Part model, mm, in its own coordinate system. A direction names the side the tool comes from. Give positions to 0.01 mm unless a question says otherwise; leave off trailing zeros. Write each loop counter-clockwise with the first axis right and the second up, starting at its lowest first coordinate (ties: lowest second). Pieces come first, ordered by that corner, then holes.
from build123d import *

# Parameters (mm, degrees)
SKETCH_1_R          = 1.025
EXTRUDE_1_DEPTH     = 2.5
EXTRUDE_3_DEPTH     = 2.5
EXTRUDE_2_DEPTH     = 2.5
FILLET_1_R          = 4
CUT_EXTRUDE_1_DEPTH = 2.5
FILLET_3_R          = 1
FILLET_4_R          = 2


with BuildPart() as part:
    # 草图1 → 凸台-拉伸1 (new body)
    with BuildSketch(Plane(origin=(0, 0, 0), x_dir=(1, 0, 0), z_dir=(0, 1, 0))):
        with BuildLine():
            Line((0, 4), (30, 4))
            ThreePointArc((30, 4), (34, 0), (30, -4))
            Line((30, -4), (0, -4))
            ThreePointArc((0, -4), (-4, 0), (0, 4))
        make_face()
        with Locations(Location((30, 0, 0), (0, 0, 270))):
            Circle(SKETCH_1_R, mode=Mode.SUBTRACT)
        with BuildLine():
            Line((0, 1.6), (20, 1.6))
            ThreePointArc((20, 1.6), (21.6, 0), (20, -1.6))
            Line((20, -1.6), (0, -1.6))
            ThreePointArc((0, -1.6), (-1.6, 0), (0, 1.6))
        make_face(mode=Mode.SUBTRACT)
    extrude(amount=EXTRUDE_1_DEPTH)

    # 草图4 → 凸台-拉伸3 (add)
    with BuildSketch(Plane(origin=(0, 0, 0), x_dir=(1, 0, 0), z_dir=(0, 1, 0))):
        with BuildLine():
            Line((35, 4), (30, 4))
            ThreePointArc((30, 4), (34, 0), (30, -4))
            Line((30, -4), (35, -4))
            Line((35, -4), (35, 4))
        make_face()
    extrude(amount=EXTRUDE_3_DEPTH)

    # 草图2 → 凸台-拉伸2 (add)
    with BuildSketch(Plane.XZ):
        with BuildLine():
            Line((-4, 6.7), (-4, 0))
            ThreePointArc((-4, 0), (-2.828427125, 2.828427125), (0, 4))
            Line((0, 4), (33.541672043, 4))
            ThreePointArc((33.541672043, 4), (33.13675384, 5.32310053), (33, 6.7))
            ThreePointArc((33, 6.7), (14.5, 5.554795019), (-4, 6.7))
        make_face()
    extrude(amount=-EXTRUDE_2_DEPTH)

    # 圆角1
    fillet_1_edges = [part.edges().sort_by_distance(p)[0] for p in [
        (-4, 1.25, 6.7),
    ]]
    fillet(fillet_1_edges, radius=FILLET_1_R)

    # 草图5 → 切除-拉伸1 (cut)
    with BuildSketch(Plane(origin=(0, 2.5, 0), x_dir=(1, 0, 0), z_dir=(0, 1, 0))):
        with BuildLine():
            ThreePointArc((34.376520653, 0), (34.165583782, -2.043096437), (33.541672043, -4))
            Line((33.541672043, -4), (35, -4))
            Line((35, -4), (35, 4))
            Line((35, 4), (33.541672043, 4))
            ThreePointArc((33.541672043, 4), (34.165583782, 2.043096437), (34.376520653, 0))
        make_face()
    extrude(amount=-CUT_EXTRUDE_1_DEPTH, mode=Mode.SUBTRACT)

    # 圆角3
    fillet_3_edges = [part.edges().sort_by_distance(p)[0] for p in [
        (33, 1.25, 6.7),
    ]]
    fillet(fillet_3_edges, radius=FILLET_3_R)

    # 圆角4
    fillet_4_edges = [part.edges().sort_by_distance(p)[0] for p in [
        (33.541672043, 1.25, -4),
    ]]
    fillet(fillet_4_edges, radius=FILLET_4_R)


solid = part.part
1) Flat gauge pins, fed straight in: P1, Ø1.2, axis at x = 11.5, y = 1, coming from the +Z side; P2, Ø2.5, axis at x = 30, z = 0, coming from the +Y side. Where does each tip first touch, or does it go through?
Check result:
P1: stops at z = 5.6
P2: stops at y = 2.5
2) Saw through at A-A (x = 30). Write the cut outline in (y, z) (3 decimals).
Check result:
outline: (0, -4) - (2.5, -4) - (2.5, -1.025) - (0, -1.025) - close; (0, 1.025) - (2.5, 1.025) - (2.5, 6.358) - (0, 6.358) - close
3) Saw through at C-C (x = 22). Write the cut outline in (y, z), and give its area (3 significant figures).
Check result:
outline: (0, -4) - (2.5, -4) - (2.5, 5.74) - (0, 5.74) - close
area: 24.4 mm2
4) Saw through at B-B (y = 1.6). State how many separate pieces and enclosed holes the cut face has, and give its area (3 significant figures).
Check result:
separate pieces: 1
enclosed holes: 2
area: 293 mm2
5) 3-axis set-ups, long thin cutter, end or side, ignore diameter. For faces 4 (the cylindrical face through (21.6, 1.2, 0)), 5 (the cylindrical face through (-2.859, 1.232, -2.797)): which of +Z, -Z, +X, -X, +Y, -Y reach the whole face in a straight line?
Check result:
face 4: +Y, -Y
face 5: -Z, -X, +Y, -Y
6) Drill centre lines: L1, parallel to Z at x = 8, y = 0.25; L2, parallel to Z at x = 31.5, y = 1.7; L3, parallel to X at y = 0.9, z = -3. Where is each one in solid material? Low to high.
Check result:
L1: z = -4 to -1.6, 1.6 to 5.7
L2: z = -4 to 6.52
L3: x = -2.65 to 33.85
7) Mould opens along X. For faces 1 (the cylindrical face through (-1.6, 1.2, 0)), 2 (the cylindrical face through (33.253, 1.232, 4.833)), 3 (the flat face through (15, 0, 3)) say: +X half, -X half, draft (parallel to the pull), parting line (faces both ways), or undercut.
Check result:
face 1: undercut
face 2: +X half
face 3: draft
